CAD build for the part. Positions are in the model's coordinates, mm. Face numbers are marked on the shaded views. A direction names the side the tool comes from. Coordinates: 2 decimals unless noted, no trailing zeros. Order: outer loops, then holes, each group sorted by start corner. A loop starts at its lowest first (then second) coordinate and runs counter-clockwise, first axis right, second up. Notation, with made-up numbers: M -25.75,16 L 4.25,16 A14 ccw 4.25,30 Z; hole C 19.5,-3 d2. An arc over 180 degrees is marked long. Write item = value, one per line.
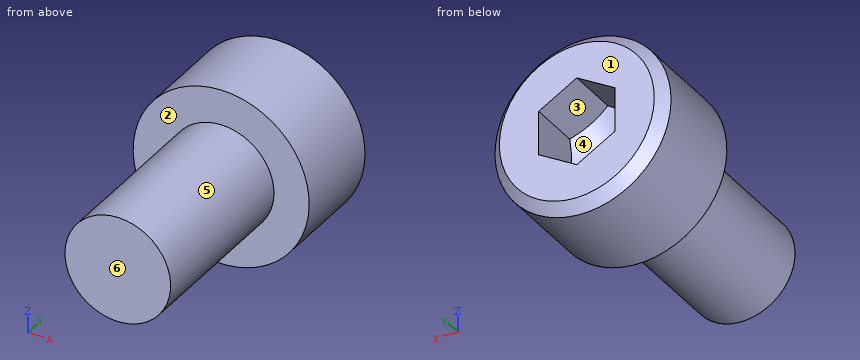
from build123d import *

# Parameters (mm, degrees)
CROQUIS4_R              = 5
SALIENTE_EXTRUIR3_DEPTH = 6
CHAFL_N2_SIZE           = 0.6
CROQUIS6_5_R            = 3
SALIENTE_EXTRUIR7_DEPTH = 10


with BuildPart() as part:
    # Croquis4 → Saliente-Extruir3 (new body)
    with BuildSketch(Plane(origin=(0, 0, 0), x_dir=(1, 0, 0), z_dir=(0, 1, 0))):
        with Locations(Location((0, 0, 0), (0, 0, 270))):
            Circle(CROQUIS4_R)
        Polygon((0, 2.5), (-2.165063509, 1.25), (-2.165063509, -1.25), (0, -2.5), (2.165063509, -1.25), (2.165063509, 1.25), align=None, mode=Mode.SUBTRACT)
    extrude(amount=SALIENTE_EXTRUIR3_DEPTH)

    # Chafl_n2
    chafl_n2_edges = [part.edges().sort_by_distance(p)[0] for p in [
        (0, 6, -5),
    ]]
    chamfer(chafl_n2_edges, length=CHAFL_N2_SIZE)

    # Croquis5 → Revoluci_n2 (revolve)
    with BuildSketch(Plane.XY, mode=Mode.PRIVATE) as revoluci_n2_sk:
        Polygon((0, 0), (0, 1.556624327), (2.5, 3), (5, 3), (5, 0), align=None)
    revolve(revoluci_n2_sk.sketch.rotate(Axis((0, 0, 0), (0, 1, 0)), 90), axis=Axis((0, 0, 0), (0, 1, 0)))

    # Croquis6_5 → Saliente-Extruir7 (add)
    with BuildSketch(Plane.XZ):
        with Locations(Location((0, 0, 0), (0, 0, 90))):
            Circle(CROQUIS6_5_R)
    extrude(amount=SALIENTE_EXTRUIR7_DEPTH)


solid = part.part
(1) Wall check: line 1 (Z direction, x = -1, y = 3.5); line 2 (Y direction, x = 3, z = 2.75); line 3 (Z direction, x = -0.75, y = 4.25). Give the ranges that are in metal, low to high. Write a range as from..to.
Evaluation:
line_1 = -4.9..-1.92, 1.92..4.9
line_2 = 0..6
line_3 = -4.94..-2.07, 2.07..4.94
(2) Tool access for the marked faces 1, 2 and 3: list every direction of +Z, -Z, +X, -X, +Y, -Y with a clear straight run to the whole face (end or side of a thin tool).
Evaluation:
face_1 = +Z, -Z, +X, -X, +Y
face_2 = -Y
face_3 = +Y
(3) Slice it at B-B, the plane y = -7. Write the cut outline in (x, z).
Evaluation:
outline = C 0,0 d6
(4) Slice it at A-A, the plane y = 4.5. Write the cut outline in (x, z).
Evaluation:
outline = C 0,0 d10; hole M -2.17,-1.25 L 0,-2.5 L 2.17,-1.25 L 2.17,1.25 L 0,2.5 L -2.17,1.25 Z
(5) Pin check, flat tips, straight feed: pin 1 Ø5 at (x, y) = (3.5, 0) entering from +Z; pin 2 Ø1.5 at (x, y) = (3.5, -8) entering from +Z; pin 3 Ø1 at (x, y) = (3, -2) entering from -Z. Stop position of each tip, or through.
Evaluation:
pin_1 = 4.9
pin_2 = 1.2
pin_3 = -1.66
(6) Pull direction X, two halves, no side cores. Call the marked faces 4, 5 and 6: +X half, -X half, draft (parallel to the pull), parting line (faces both ways), or undercut.
Evaluation:
face_4 = undercut
face_5 = parting line
face_6 = draft
